For this review, take the finished solid that the model builds, in its own axes (mm). A direction names the side the tool comes from. Coordinates: 2 decimals unless noted, no trailing zeros. Write each loop counter-clockwise with the first axis right and the second up, starting at its lowest first coordinate (ties: lowest second). Pieces come first, ordered by that corner, then holes.
```python
from build123d import *

# Parameters (mm, degrees)
SKETCH1_R           = 2.53125
BOSS_EXTRUDE1_DEPTH = 6.35
SKETCH2_R           = 1.1684
CUT_EXTRUDE1_DEPTH  = 6.35


with BuildPart() as part:
    # Sketch1 → Boss-Extrude1 (new body)
    with BuildSketch(Plane.XY):
        with BuildLine():
            Line((-6, 0), (-6, -2.2225))
            Line((-6, -2.2225), (-11.08, -2.2225))
            Line((-11.08, -2.2225), (-11.08, -6.985))
            Line((-11.08, -6.985), (11.08, -6.985))
            Line((11.08, -6.985), (11.08, -2.2225))
            Line((11.08, -2.2225), (6, -2.2225))
            Line((6, -2.2225), (6, 0))
            ThreePointArc((6, 0), (0, 6), (-6, 0))
        make_face()
        Circle(SKETCH1_R, mode=Mode.SUBTRACT)
    extrude(amount=BOSS_EXTRUDE1_DEPTH)

    # Sketch2 → Cut-Extrude1 (cut)
    with BuildSketch(Plane(origin=(0, -2.2225, 0), x_dir=(1, 0, 0), z_dir=(0, 1, 0))):
        with Locations(Location((-8.54, -3.175, 0), (0, 0, 270))):
            Circle(SKETCH2_R)
        with Locations(Location((8.54, -3.175, 0), (0, 0, 270))):
            Circle(SKETCH2_R)
    extrude(amount=-CUT_EXTRUDE1_DEPTH, mode=Mode.SUBTRACT)


solid = part.part
```
1) For L1, parallel to X at y = -6, z = 3.25; L2, parallel to X at y = -4.25, z = 2.5; L3, parallel to Y at x = -1.75, z = 1 (3 decimals), list the stretches that pass through material, from the lowest coordinate up.
2) The part is to be moulded in two halves that separate along X. For faces 4 (the face through (11.08, -5, 3)), 5 (the face through (1.361, 2.134, 3.131)), 6 (the face through (-11.08, -5, 3)), say which applies: pulls with the +X half, pulls with the -X half, needs draft (parallel to the pull), parting line crosses it, or undercut.
3) Consider section C-C (y = 0.5). Give the boundary of the cut face in (x, z).
4) Clearance check with a flat-ended pin moving along its axis: P1, Ø1.5, axis at x = -9, z = 2.5, coming from the +Y side. State where the tip first meets the part, or that it passes through.
5) Tool access review of faces 1 (the face through (10, -2.222, 4)), 2 (the face through (0, -3, 6.35)), 3 (the face through (-6, -1, 3)): name each direction out of +Z, -Z, +X, -X, +Y, -Y from which nothing blocks a thin tool from reaching the whole face with its end or side.
6) Consider section D-D (x = -4). Give the boundary of the cut face in (y, z) (3 decimals), then the cut area to 3 significant figures.
7) Consider section B-B (z = 5.25). Give the boundary of the cut face in (x, y) (1 decimal), then the cut area to 3 significant figures.
Results:
1. L1: x = -11.08 to -9.71, -7.37 to 7.37, 9.71 to 11.08
1. L2: x = -11.08 to -9.49, -7.59 to 7.59, 9.49 to 11.08
1. L3: y = -6.985 to -1.829, 1.829 to 5.739
2. face 4: pulls with the +X half
2. face 5: undercut
2. face 6: pulls with the -X half
3. outline: (-5.98, 0) - (-2.48, 0) - (-2.48, 6.35) - (-5.98, 6.35) - close; (2.48, 0) - (5.98, 0) - (5.98, 6.35) - (2.48, 6.35) - close
4. P1: stops at y = -2.22
5. face 1: +Z, -Z, +X, +Y
5. face 2: +Z, +X, -X, +Y, -Y
5. face 3: +Z, -Z, -X, +Y
6. outline: (-6.985, 0) - (4.472, 0) - (4.472, 6.35) - (-6.985, 6.35) - close
6. area: 72.8 mm2
7. outline: (-11.1, -7) - (11.1, -7) - (11.1, -2.2) - (6, -2.2) - (6, 0) arc R6 ccw to (-6, 0) - (-6, -2.2) - (-11.1, -2.2) - close; hole circle Ø5.1 at (0, 0)
7. area: 169 mm2
